Can you work these out from the model? Positions are in its coordinate system, mm. A direction names the side the tool comes from. Give positions to 0.01 mm unless a question says otherwise; leave off trailing zeros. Loops run counter-clockwise (first coordinate to the right, second up) from the corner with the lowest first, then second, coordinate; pieces in that order, holes last. Notation, with made-up numbers: (48, -31) - (102, -31) arc R36 cw to (102, 3) - close; hole circle Ø5 at (26, 49). An arc over 180 degrees is marked (long way). Use a Markdown table: item, result. Add a question column.
```python
from build123d import *

# Parameters (mm, degrees)
SKETCH1_W                    = 190
SKETCH1_H                    = 105
BASE_FLANGE1_DEPTH           = 1.5
EDGE_FLANGE1_STRIP_W         = 7.4732
EDGE_FLANGE1_STRIP_H         = 1.5
EDGE_FLANGE1_STRIP_CUT_DEPTH = 190
EDGE_FLANGE1_DEPTH           = 190
SKETCH9_R                    = 3.004998415
CUT_EXTRUDE1_DEPTH           = 10
LPATTERN1_COUNT              = 3
LPATTERN1_PITCH              = 75


# Sheet-metal steps are written as plain solids
with BuildPart() as part:
    # Sketch1 → Base-Flange1 (new body)
    with BuildSketch(Plane.XY):
        with Locations((-7.105263158, -3.728070175)):
            Rectangle(SKETCH1_W, SKETCH1_H)
    extrude(amount=-BASE_FLANGE1_DEPTH)

    # Edge-Flange1 strip (across the edge) → Edge-Flange1 strip cut (cut)
    with BuildSketch(Plane(origin=(87.894736842, 48.771929825, 0), x_dir=(0, -1, 0), z_dir=(-1, 0, 0))):
        with Locations((-1.5, -0.75)):
            Rectangle(EDGE_FLANGE1_STRIP_W, EDGE_FLANGE1_STRIP_H)
    extrude(amount=EDGE_FLANGE1_STRIP_CUT_DEPTH, mode=Mode.SUBTRACT)

    # Edge-Flange1 section (across the edge) → Edge-Flange1 (add)
    with BuildSketch(Plane(origin=(87.894736842, 48.771929825, 0), x_dir=(0, -1, 0), z_dir=(-1, 0, 0))):
        with BuildLine():
            Line((0, 0.7366), (0, 18.5))
            Line((0, 18.5), (1.5, 18.5))
            Line((1.5, 18.5), (1.5, 0.7366))
            ThreePointArc((1.5, 0.7366), (1.715745145, 0.215745145), (2.2366, 0))
            Line((2.2366, 0), (2.2366, -1.5))
            ThreePointArc((2.2366, -1.5), (0.655084973, -0.844915027), (0, 0.7366))
        make_face()
    extrude(amount=EDGE_FLANGE1_DEPTH)

    # Sketch9 → Cut-Extrude1 (cut)
    with BuildSketch(Plane.XZ.offset(-47.271929825)):
        with Locations(Location((-77.977994627, 9.946382275, 0), (0, 0, 270))):
            Circle(SKETCH9_R)
    cut_extrude1 = extrude(amount=-CUT_EXTRUDE1_DEPTH, mode=Mode.SUBTRACT)

    # LPattern1: Cut-Extrude1 ×3
    with Locations(*[(i * LPATTERN1_PITCH, 0, 0) for i in range(1, LPATTERN1_COUNT)]):
        add(cut_extrude1, mode=Mode.SUBTRACT)


solid = part.part
```
1. Please list where these lines run through material, in increasing order: line 1 along Z through (x, y) = (58, 22.5); line 2 along Y through (x, z) = (27, 11.25); line 3 along Y through (x, z) = (36, 0.5). Write a range as [from, to].
2. Will these pins go through, and if not, where does the flat tip stop? P1, Ø5.5, axis at x = 18, z = 6, coming from the -Y side; P2, Ø5, axis at x = -58, y = 15.5, coming from the +Z side; P3, Ø7, axis at x = -77.98, z = 9.95, coming from the +Y side; P4, Ø3.5, axis at x = -2.98, z = 9.95, coming from the -Y side.
3. If we mould it in two halves opening along X, with no side actions, what happens to faces 1 (the face through (87.895, -4, -0.3)), 2 (the face through (-8, -4, 0)), 3 (the face through (-5.644, 48.011, 8.56))? For each: released by +X, released by -X, zero draft, split by the parting line, or undercut.
4. On a 3-axis mill with a long thin cutter (end or side, diameter ignored), from which of +Z, -Z, +X, -X, +Y, -Y can I reach the whole of each face in a straight line? I mean faces 4 (the face through (-6, 48.772, 11)), 5 (the face through (-6, 47.272, 12)). Say none if no direction works.
5. Suppose I cut it at A-A (x = 27). List the corners of the cut face in (y, z) for me, and give its area (3 significant figures).
6. Suppose I cut it at C-C (y = -12). List the corners of the cut face in (x, z) for me, and give its area (3 significant figures).
7. Suppose I cut it at B-B (z = 9.75). List the corners of the cut face in (x, y) for me, and give its area (3 significant figures).
Results below:
| question | item | result |
|---|---|---|
| 1 | line 1 | [-1.5, 0] |
| 1 | line 2 | [47.27, 48.77] |
| 1 | line 3 | [47.23, 48.76] |
| 2 | P1 | y = 47.27 |
| 2 | P2 | z = 0 |
| 2 | P3 | y = 48.77 |
| 2 | P4 | through |
| 3 | face 1 | released by +X |
| 3 | face 2 | zero draft |
| 3 | face 3 | undercut |
| 4 | face 4 | +Z, -Z, +X, -X, +Y |
| 4 | face 5 | +Z, +X, -X, -Y |
| 5 | outline | (-56.23, -1.5) - (46.54, -1.5) arc R2.24 ccw to (48.77, 0.74) - (48.77, 18.5) - (47.27, 18.5) - (47.27, 0.74) arc R0.74 cw to (46.54, 0) - (-56.23, 0) - close |
| 5 | area | 184 mm² |
| 6 | outline | (-102.11, -1.5) - (87.89, -1.5) - (87.89, 0) - (-102.11, 0) - close |
| 6 | area | 285 mm² |
| 7 | outline | (-102.11, 47.27) - (-80.98, 47.27) - (-80.98, 48.77) - (-102.11, 48.77) - close; (-74.98, 47.27) - (-5.98, 47.27) - (-5.98, 48.77) - (-74.98, 48.77) - close; (0.02, 47.27) - (69.02, 47.27) - (69.02, 48.77) - (0.02, 48.77) - close; (75.02, 47.27) - (87.89, 47.27) - (87.89, 48.77) - (75.02, 48.77) - close |
| 7 | area | 258 mm² |
